Read the model definition and answer for the solid it produces. Units are mm, in the model's axes. A direction names the side the tool comes from. Coordinates: 2 decimals unless noted, no trailing zeros. Write each loop counter-clockwise with the first axis right and the second up, starting at its lowest first coordinate (ties: lowest second). Pieces come first, ordered by that corner, then holes.
1) The part is cut by section D-D (z = -101). Determine the outline of the cut face in (x, y) (3 decimals), then the cut area to 3 significant figures.
2) This flat-tipped pin is pushed along its axis until it touches: pin 1 Ø1.5 at (x, y) = (-237.5, 368.5) entering from -Z (3 decimals). Where does it stop, or does it pass through?
3) The part is cut by section B-B (z = -33). Determine the outline of the cut face in (x, y) (3 decimals), then the cut area to 3 significant figures.
4) The part is cut by section C-C (y = -282). Determine the outline of the cut face in (x, z) (3 decimals).
5) Which of the six approach directions +Z, -Z, +X, -X, +Y, -Y give full straight-line access (tool end or side, diameter ignored) to faces 1 (the face through (-354, -482, -102)), 2 (the face through (-3.175, -8, -79))?
6) Determine the mould class of faces 3 (the face through (-355.6, -8, -75)), 4 (the face through (-352.425, -8, -79)), 5 (the face through (-141.46, 11.44, -1.57)), 6 (the face through (-353.99, 483.667, -100.889)) for opening direction X: +X half, -X half, draft (parallel to the pull), parting line (faces both ways), or undercut.
7) Find the intervals of material crossed by line 1 (X direction, y = 533.4, z = -1.55) (3 decimals); line 2 (X direction, y = 533, z = -1); line 3 (Y direction, x = -266, z = -1), in increasing order.
8) The part is cut by section A-A (y = 0). Determine the outline of the cut face in (x, z) (3 decimals).
from build123d import *

# Parameters (mm, degrees)
F0_W     = 1117.6
F0_H     = 152.4
F1_DEPTH = 355.6
F2_W     = 349.25
F2_H     = 149.225
F3_DEPTH = 1117.601
F5_DEPTH = 355.601
F6_R     = 38.1
F6_R_2   = 3.175
F7_DEPTH = 152.401


with BuildPart() as f1:
    # F0 (on Right) → F1 (new body)
    with BuildSketch(Plane.YZ):
        with Locations((0, -76.2)):
            Rectangle(F0_W, F0_H)
    extrude(amount=-F1_DEPTH)

    # F2 (on face) → F3 (cut, through all)
    with BuildSketch(Plane.XZ.offset(558.8)):
        with Locations((-177.8, -77.7875)):
            Rectangle(F2_W, F2_H)
    extrude(amount=-F3_DEPTH, mode=Mode.SUBTRACT)

    # F4 (on face) → F5 (cut, through all)
    with BuildSketch(Plane.YZ):
        Polygon((-406.4, -152.4), (-558.8, -50.8), (-558.8, -152.4), align=None)
        Polygon((558.8, -152.4), (558.8, -50.8), (406.4, -152.4), align=None)
    extrude(amount=-F5_DEPTH, mode=Mode.SUBTRACT)

    # F6 (on face) → F7 (cut, through all)
    with BuildSketch(Plane.XY):
        with Locations((-177.8, 0)):
            Circle(F6_R)
        with Locations((-12.7, 203.2)):
            Circle(F6_R_2)
        with Locations((-266.7, 203.2)):
            Circle(F6_R_2)
        with Locations((-266.7, 533.4)):
            Circle(F6_R_2)
        with Locations((-12.7, 533.4)):
            Circle(F6_R_2)
        with Locations((-76.2, -355.6)):
            Circle(F6_R_2)
        with Locations((-76.2, -152.4)):
            Circle(F6_R_2)
        with Locations((-279.4, -152.4)):
            Circle(F6_R_2)
        with Locations((-279.4, -355.6)):
            Circle(F6_R_2)
    extrude(amount=-F7_DEPTH, mode=Mode.SUBTRACT)


solid = f1.part
Reported:
1. outline: (-355.6, -483.5) - (-352.425, -483.5) - (-352.425, 483.5) - (-355.6, 483.5) - close; (-3.175, -483.5) - (0, -483.5) - (0, 483.5) - (-3.175, 483.5) - close
1. area: 6,140 mm2
2. pin 1: stops at z = -3.175
3. outline: (-355.6, -558.8) - (-352.425, -558.8) - (-352.425, 558.8) - (-355.6, 558.8) - close; (-3.175, -558.8) - (0, -558.8) - (0, 558.8) - (-3.175, 558.8) - close
3. area: 7,100 mm2
4. outline: (-355.6, -152.4) - (-352.425, -152.4) - (-352.425, -3.175) - (-3.175, -3.175) - (-3.175, -152.4) - (0, -152.4) - (0, 0) - (-355.6, 0) - close
5. face 1: -Z, +X, -X, -Y
5. face 2: -Z, +Y, -Y
6. face 3: -X half
6. face 4: undercut
6. face 5: undercut
6. face 6: draft
7. line 1: x = -355.6 to -269.875, -263.525 to -15.875, -9.525 to 0
7. line 2: x = -355.6 to -269.85, -263.55 to -15.85, -9.55 to 0
7. line 3: y = -558.8 to 200.1, 206.3 to 530.3, 536.5 to 558.8
8. outline: (-355.6, -152.4) - (-352.425, -152.4) - (-352.425, -3.175) - (-215.9, -3.175) - (-215.9, 0) - (-355.6, 0) - close; (-139.7, -3.175) - (-3.175, -3.175) - (-3.175, -152.4) - (0, -152.4) - (0, 0) - (-139.7, 0) - close
